```python
from build123d import *

# Parameters (mm, degrees)
F0_R     = 2.4892
F1_DEPTH = 1.5875
F2_R     = 6.35


with BuildPart() as f1:
    # F0 (on Top) → F1 (new body, symmetric)
    with BuildSketch(Plane.XY):
        Polygon((-38.1, 12.7), (-38.1, -12.7), (38.1, -12.7), (38.1, 12.7), (12.7, 12.7), (12.7, 63.5), (-12.7, 63.5), (-12.7, 12.7), align=None)
        with Locations((-25.4, 0)):
            Circle(F0_R, mode=Mode.SUBTRACT)
        Circle(F0_R, mode=Mode.SUBTRACT)
        with Locations((25.4, 0)):
            Circle(F0_R, mode=Mode.SUBTRACT)
        with Locations((0, 25.4)):
            Circle(F0_R, mode=Mode.SUBTRACT)
        with Locations((0, 50.8)):
            Circle(F0_R, mode=Mode.SUBTRACT)
    extrude(amount=F1_DEPTH, both=True)

    # F2
    f2_edges = [f1.edges().sort_by_distance(p)[0] for p in [
        (-12.7, 12.7, 0),
        (-12.7, 63.5, 0),
        (12.7, 63.5, 0),
        (12.7, 12.7, 0),
        (38.1, 12.7, 0),
        (38.1, -12.7, 0),
        (-38.1, -12.7, 0),
        (-38.1, 12.7, 0),
    ]]
    fillet(f2_edges, radius=F2_R)


solid = f1.part
```
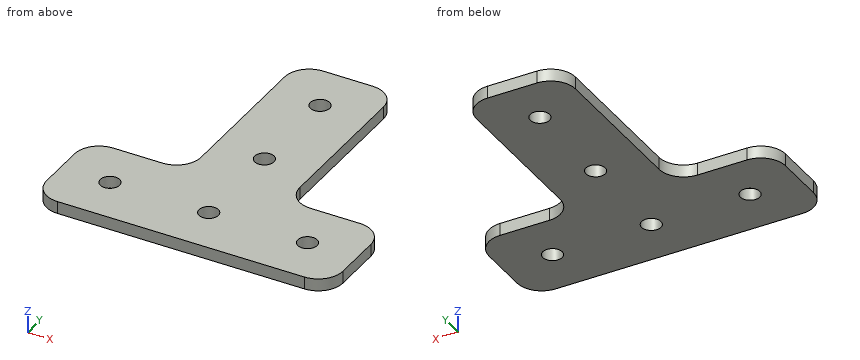
Can you work these out from the model? Positions are in its coordinate system, mm. Round coordinates to 2 decimals unless told otherwise and drop trailing zeros. Loops run counter-clockwise (first coordinate to the right, second up) from the corner with the lowest first, then second, coordinate; pieces in that order, holes last.
Item 1: Suppose I cut it at A-A, the plane x = 0. Write out the boundary of the cut face in (y, z), then the cut area to 3 significant figures.
Item 2: Suppose I cut it at C-C, the plane z = -0.95. Write out the boundary of the cut face in (x, y).
Item 3: Suppose I cut it at D-D, the plane y = 0. Write out the boundary of the cut face in (x, z), then the cut area to 3 significant figures.
Item 4: Please list where these lines run through material, in increasing order: L1, parallel to Y at x = 0, z = -0.05; L2, parallel to Y at x = 25.4, z = 0.7; L3, parallel to X at y = 1, z = 0.5.
Item 5: Will these pins go through, and if not, where does the flat tip stop? pin 1 Ø6.5 at (x, y) = (-25.4, 0) entering from +Z; pin 2 Ø1.6 at (x, z) = (28, 0.5) entering from +Y; pin 3 Ø4.5 at (x, y) = (0, 50.8) entering from +Z; pin 4 Ø1.5 at (y, z) = (18, -1) entering from -X.
Item 6: Suppose I cut it at B-B, the plane y = 50.8. Write out the boundary of the cut face in (x, z), then the cut area to 3 significant figures.
Reported:
1. outline: (-12.7, -1.59) - (-2.49, -1.59) - (-2.49, 1.59) - (-12.7, 1.59) - close; (2.49, -1.59) - (22.91, -1.59) - (22.91, 1.59) - (2.49, 1.59) - close; (27.89, -1.59) - (48.31, -1.59) - (48.31, 1.59) - (27.89, 1.59) - close; (53.29, -1.59) - (63.5, -1.59) - (63.5, 1.59) - (53.29, 1.59) - close
1. area: 195 mm2
2. outline: (-38.1, -6.35) arc R6.35 ccw to (-31.75, -12.7) - (31.75, -12.7) arc R6.35 ccw to (38.1, -6.35) - (38.1, 6.35) arc R6.35 ccw to (31.75, 12.7) - (19.05, 12.7) arc R6.35 cw to (12.7, 19.05) - (12.7, 57.15) arc R6.35 ccw to (6.35, 63.5) - (-6.35, 63.5) arc R6.35 ccw to (-12.7, 57.15) - (-12.7, 19.05) arc R6.35 cw to (-19.05, 12.7) - (-31.75, 12.7) arc R6.35 ccw to (-38.1, 6.35) - close; hole circle Ø4.98 at (-25.4, 0); hole circle Ø4.98 at (0, 0); hole circle Ø4.98 at (0, 25.4); hole circle Ø4.98 at (0, 50.8); hole circle Ø4.98 at (25.4, 0)
3. outline: (-38.1, -1.59) - (-27.89, -1.59) - (-27.89, 1.59) - (-38.1, 1.59) - close; (-22.91, -1.59) - (-2.49, -1.59) - (-2.49, 1.59) - (-22.91, 1.59) - close; (2.49, -1.59) - (22.91, -1.59) - (22.91, 1.59) - (2.49, 1.59) - close; (27.89, -1.59) - (38.1, -1.59) - (38.1, 1.59) - (27.89, 1.59) - close
3. area: 195 mm2
4. L1: y = -12.7 to -2.49, 2.49 to 22.91, 27.89 to 48.31, 53.29 to 63.5
4. L2: y = -12.7 to -2.49, 2.49 to 12.7
4. L3: x = -38.1 to -27.68, -23.12 to -2.28, 2.28 to 23.12, 27.68 to 38.1
5. pin 1: stops at z = 1.59
5. pin 2: stops at y = 12.7
5. pin 3: passes through
5. pin 4: stops at x = -12.96
6. outline: (-12.7, -1.59) - (-2.49, -1.59) - (-2.49, 1.59) - (-12.7, 1.59) - close; (2.49, -1.59) - (12.7, -1.59) - (12.7, 1.59) - (2.49, 1.59) - close
6. area: 64.8 mm2
